from build123d import *

# Parameters (mm, degrees)
SKETCH1_R           = 15.3924
BOSS_EXTRUDE1_DEPTH = 0.508


with BuildPart() as part:
    # Sketch1 → Boss-Extrude1 (new body)
    with BuildSketch(Plane(origin=(0, 0, 0), x_dir=(1, 0, 0), z_dir=(0, 1, 0))):
        Circle(SKETCH1_R)
        with BuildLine():
            Line((-1.524, 14.269850209), (-0.762, 13.822011612))
            ThreePointArc((-0.762, 13.822011612), (0, 13.843), (0.762, 13.822011612))
            Line((0.762, 13.822011612), (1.524, 14.269850209))
            ThreePointArc((1.524, 14.269850209), (3.714312116, 13.862001533), (5.815102389, 13.12005279))
            Line((5.815102389, 13.12005279), (6.251094448, 12.351213187))
            ThreePointArc((6.251094448, 12.351213187), (6.9215, 11.988389665), (7.570917164, 11.589213187))
            Line((7.570917164, 11.589213187), (8.45474782, 11.59605279))
            ThreePointArc((8.45474782, 11.59605279), (10.147689417, 10.147689417), (11.59605279, 8.45474782))
            Line((11.59605279, 8.45474782), (11.589213187, 7.570917164))
            ThreePointArc((11.589213187, 7.570917164), (11.988389665, 6.9215), (12.351213187, 6.251094448))
            Line((12.351213187, 6.251094448), (13.12005279, 5.815102389))
            ThreePointArc((13.12005279, 5.815102389), (13.862001533, 3.714312116), (14.269850209, 1.524))
            Line((14.269850209, 1.524), (13.822011612, 0.762))
            ThreePointArc((13.822011612, 0.762), (13.843, 0), (13.822011612, -0.762))
            Line((13.822011612, -0.762), (14.269850209, -1.524))
            ThreePointArc((14.269850209, -1.524), (13.862001533, -3.714312116), (13.12005279, -5.815102389))
            Line((13.12005279, -5.815102389), (12.351213187, -6.251094448))
            ThreePointArc((12.351213187, -6.251094448), (11.988389665, -6.9215), (11.589213187, -7.570917164))
            Line((11.589213187, -7.570917164), (11.59605279, -8.45474782))
            ThreePointArc((11.59605279, -8.45474782), (10.147689417, -10.147689417), (8.45474782, -11.59605279))
            Line((8.45474782, -11.59605279), (7.570917164, -11.589213187))
            ThreePointArc((7.570917164, -11.589213187), (6.9215, -11.988389665), (6.251094448, -12.351213187))
            Line((6.251094448, -12.351213187), (5.815102389, -13.12005279))
            ThreePointArc((5.815102389, -13.12005279), (3.714312116, -13.862001533), (1.524, -14.269850209))
            Line((1.524, -14.269850209), (0.762, -13.822011612))
            ThreePointArc((0.762, -13.822011612), (0, -13.843), (-0.762, -13.822011612))
            Line((-0.762, -13.822011612), (-1.524, -14.269850209))
            ThreePointArc((-1.524, -14.269850209), (-3.714312116, -13.862001533), (-5.815102389, -13.12005279))
            Line((-5.815102389, -13.12005279), (-6.251094448, -12.351213187))
            ThreePointArc((-6.251094448, -12.351213187), (-6.9215, -11.988389665), (-7.570917164, -11.589213187))
            Line((-7.570917164, -11.589213187), (-8.45474782, -11.59605279))
            ThreePointArc((-8.45474782, -11.59605279), (-10.147689417, -10.147689417), (-11.59605279, -8.45474782))
            Line((-11.59605279, -8.45474782), (-11.589213187, -7.570917164))
            ThreePointArc((-11.589213187, -7.570917164), (-11.988389665, -6.9215), (-12.351213187, -6.251094448))
            Line((-12.351213187, -6.251094448), (-13.12005279, -5.815102389))
            ThreePointArc((-13.12005279, -5.815102389), (-13.862001533, -3.714312116), (-14.269850209, -1.524))
            Line((-14.269850209, -1.524), (-13.822011612, -0.762))
            ThreePointArc((-13.822011612, -0.762), (-13.843, 0), (-13.822011612, 0.762))
            Line((-13.822011612, 0.762), (-14.269850209, 1.524))
            ThreePointArc((-14.269850209, 1.524), (-13.862001533, 3.714312116), (-13.12005279, 5.815102389))
            Line((-13.12005279, 5.815102389), (-12.351213187, 6.251094448))
            ThreePointArc((-12.351213187, 6.251094448), (-11.988389665, 6.9215), (-11.589213187, 7.570917164))
            Line((-11.589213187, 7.570917164), (-11.59605279, 8.45474782))
            ThreePointArc((-11.59605279, 8.45474782), (-10.147689417, 10.147689417), (-8.45474782, 11.59605279))
            Line((-8.45474782, 11.59605279), (-7.570917164, 11.589213187))
            ThreePointArc((-7.570917164, 11.589213187), (-6.9215, 11.988389665), (-6.251094448, 12.351213187))
            Line((-6.251094448, 12.351213187), (-5.815102389, 13.12005279))
            ThreePointArc((-5.815102389, 13.12005279), (-3.714312116, 13.862001533), (-1.524, 14.269850209))
        make_face(mode=Mode.SUBTRACT)
    extrude(amount=BOSS_EXTRUDE1_DEPTH)


solid = part.part
Build history of the part. All positions in model axes, mm. A direction names the side the tool comes from. Round coordinates to 2 decimals unless told otherwise and drop trailing zeros. Write each loop counter-clockwise with the first axis right and the second up, starting at its lowest first coordinate (ties: lowest second). Pieces come first, ordered by that corner, then holes. Notation, with made-up numbers: M 53.5,38.25 L 80.5,38.25 A20 cw 80.5,77.25 Z; hole C 27,84.25 d10. An arc over 180 degrees is marked long. Answer in a Markdown table with one row per item.
1. Mould opens along Z. For faces 1 (the face through (10.17, 0.25, 10.126)), 2 (the face through (-3.337, 0.25, 15.026)), 3 (the face through (6.8, 0, 12.5)) say: +Z half, -Z half, draft (parallel to the pull), parting line (faces both ways), or undercut.
Geometry check:
| item | result |
|---|---|
| face 1 | undercut |
| face 2 | parting line |
| face 3 | draft |
2. Probe L1, parallel to Z at x = -9, y = 0.45; L2, parallel to X at y = 0.1, z = -2; L3, parallel to Z at x = 3, y = 0.45. List the from-to ranges inside material, lowest first. Write a range as [from, to].
Geometry check:
| item | result |
|---|---|
| L1 | [-12.49, -11.18], [11.18, 12.49] |
| L2 | [-15.26, -14.21], [14.21, 15.26] |
| L3 | [-15.1, -14.03], [14.03, 15.1] |
3. Saw through at B-B (z = 0). List the corners of the cut face in (x, y), and give its area (3 significant figures).
Geometry check:
| item | result |
|---|---|
| outline | M -15.39,0 L -13.84,0 L -13.84,0.51 L -15.39,0.51 Z; M 13.84,0 L 15.39,0 L 15.39,0.51 L 13.84,0.51 Z |
| area | 1.57 mm2 |
4. Flat gauge pin, fed straight in: P1, Ø8, axis at x = 7.5, z = -5.5, coming from the -Y side. Where does the tip first touch, or does it go through?
Geometry check:
| item | result |
|---|---|
| P1 | through |
5. Which spindle directions (+Z, -Z, +X, -X, +Y, -Y) get a long thin tool onto all of the face, cutting with end or side? Do faces 4 (the face through (6.8, 0.508, 12.5)), 5 (the face through (-3.744, 0.25, -13.854)). Say none if no direction does.
Geometry check:
| item | result |
|---|---|
| face 4 | +Z, -Z, +X, -X, +Y |
| face 5 | +Y, -Y |
6. Saw through at A-A (x = 0). List the corners of the cut face in (y, z).
Geometry check:
| item | result |
|---|---|
| outline | M 0,-15.39 L 0.51,-15.39 L 0.51,-13.84 L 0,-13.84 Z; M 0,13.84 L 0.51,13.84 L 0.51,15.39 L 0,15.39 Z |
